```python
from build123d import *

# Parameters (mm, degrees)
F3_W     = 28.2
F3_H     = 38.2
F4_DEPTH = 0.5


with BuildPart() as f2:
    # F2: sweep along a path in F0
    with BuildLine(Plane.XY) as f2_path:
        Line((-12.5, 17.5), (-12.5, -17.5))
        Line((-12.5, -17.5), (12.5, -17.5))
        Line((12.5, -17.5), (12.5, 17.5))
        Line((12.5, 17.5), (-12.5, 17.5))
    # F1 (on Front) → F2 (sweep)
    with BuildSketch(Plane.XZ):
        Polygon((-14.1, 0), (-12.5, 0), (-12.5, 0.8), (-13.3, 0.8), (-13.3, 1.6), (-14.1, 1.6), align=None)
    sweep(path=f2_path.line, transition=Transition.RIGHT)

    # F3 (on face) → F4 (join)
    with BuildSketch(Plane(origin=(0, 0, 0), x_dir=(1, 0, 0), z_dir=(0, 0, -1))):
        Rectangle(F3_W, F3_H)
    extrude(amount=F4_DEPTH)


solid = f2.part
```
Could you check a few things on this model? Use its own coordinates, in mm. A direction names the side the tool comes from. Coordinates: 2 decimals unless noted, no trailing zeros. Loops run counter-clockwise (first coordinate to the right, second up) from the corner with the lowest first, then second, coordinate; pieces in that order, holes last. Notation, with made-up numbers: M 50.5,-4.75 L 78.5,-4.75 A34 ccw 78.5,30.25 Z; hole C 75.5,59.5 d8. An arc over 180 degrees is marked long. Put each result on its own line as item: value. Start each with the question number.
(1) Will these pins go through, and if not, where does the flat tip stop? P1, Ø6, axis at x = -10, y = -15, coming from the +Z side; P2, Ø8, axis at x = 6.5, y = 2, coming from the +Z side.
(2) Suppose I cut it at A-A on x = 9. Please give me the cut outline in (y, z).
(3) Thinking about a two-plate mould opening in X: for faces 3 (the face through (0, 0, 0)), 4 (the face through (-14.1, 0, 1)), 5 (the face through (0, 0, -0.5)), which applies, pulls with the +X half, pulls with the -X half, needs draft (parallel to the pull), parting line crosses it, or undercut?
(4) I need wall thicknesses on line 1 (Y direction, x = -6.5, z = 0.2); line 2 (X direction, y = -4, z = 1.1); line 3 (X direction, y = 1, z = 0.75). Which ranges of each line are inside material? Lowest first, please. Write a range as from..to.
(5) For faces 1 (the face through (0, -19.1, 1)), 2 (the face through (13, 0, 0.8)), which set-ups out of +Z, -Z, +X, -X, +Y, -Y let a thin tool reach every point of the face, with its end or its side?
(6) Suppose I cut it at B-B on y = 1. Please give me the cut outline in (x, z).
Solutions:
1. P1: stops at z = 0.8
1. P2: stops at z = 0
2. outline: M -19.1,-0.5 L 19.1,-0.5 L 19.1,1.6 L 18.3,1.6 L 18.3,0.8 L 17.5,0.8 L 17.5,0 L -17.5,0 L -17.5,0.8 L -18.3,0.8 L -18.3,1.6 L -19.1,1.6 Z
3. face 3: undercut
3. face 4: pulls with the -X half
3. face 5: needs draft
4. line 1: y = -19.1..-17.5, 17.5..19.1
4. line 2: x = -14.1..-13.3, 13.3..14.1
4. line 3: x = -14.1..-12.5, 12.5..14.1
5. face 1: +Z, -Z, +X, -X, -Y
5. face 2: +Z
6. outline: M -14.1,-0.5 L 14.1,-0.5 L 14.1,1.6 L 13.3,1.6 L 13.3,0.8 L 12.5,0.8 L 12.5,0 L -12.5,0 L -12.5,0.8 L -13.3,0.8 L -13.3,1.6 L -14.1,1.6 Z
